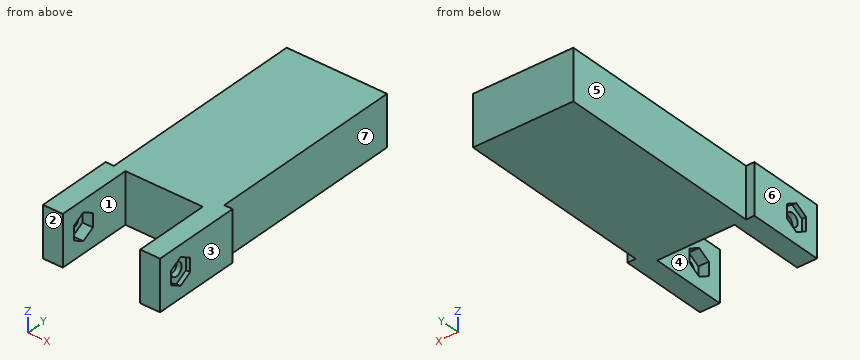
from build123d import *

# Parameters (mm, degrees)
EXTRUDE_1_DEPTH      = 12
CUT_EXTRUDE_12_DEPTH = 1
CUT_EXTRUDE_13_DEPTH = 1
CUT_EXTRUDE_14_DEPTH = 2.5
CUT_EXTRUDE_16_DEPTH = 2.5
SKETCH_26_R          = 1.55
CUT_EXTRUDE_17_DEPTH = 28


with BuildPart() as part:
    # 스케치1 → 보스-돌출1 (new body)
    with BuildSketch(Plane.XY):
        Polygon((-11.994395335, 44.774969809), (-11.994395335, -5.635030191), (-13.999795062, -5.635030191), (-13.999795062, -23.903190191), (-9.261084312, -23.903190191), (-9.261084312, -5.635030191), (9.261494188, -5.637088258), (9.261494188, -23.903190191), (14.000204938, -23.903190191), (14.000204938, -2.727088258), (12.005604665, -2.727088258), (12.005604665, 44.774969809), align=None)
    extrude(amount=EXTRUDE_1_DEPTH)

    # 스케치20 → 컷-돌출12 (cut)
    with BuildSketch(Plane(origin=(14.000204938, 0, 0), x_dir=(0, 0, -1), z_dir=(1, 0, 0))):
        Polygon((-4.384999641, -20.702278724), (-7.614999641, -20.702278724), (-9.228415158, -17.900454093), (-7.61341897, -15.106842492), (-4.380259285, -15.106842492), (-2.768420518, -17.905928971), align=None)
    extrude(amount=-CUT_EXTRUDE_12_DEPTH, mode=Mode.SUBTRACT)

    # 스케치21 → 컷-돌출13 (cut)
    with BuildSketch(Plane.ZY.offset(13.999795062)):
        Polygon((7.611047299, -20.705014823), (4.381047299, -20.705014823), (2.767631782, -17.903190191), (4.38262797, -15.109578591), (7.615787655, -15.109578591), (9.227626422, -17.90866507), align=None)
    extrude(amount=-CUT_EXTRUDE_13_DEPTH, mode=Mode.SUBTRACT)

    # 스케치22 → 컷-돌출14 (cut)
    with BuildSketch(Plane.ZY.offset(-9.261494188)):
        Polygon((7.615000359, -20.702278724), (4.385000359, -20.702278724), (2.771584842, -17.900454093), (4.38658103, -15.106842492), (7.619740715, -15.106842492), (9.231579482, -17.905928971), align=None)
    extrude(amount=-CUT_EXTRUDE_14_DEPTH, mode=Mode.SUBTRACT)

    # 스케치25 → 컷-돌출16 (cut)
    with BuildSketch(Plane(origin=(-9.261084312, 0, 0), x_dir=(0, 0, -1), z_dir=(1, 0, 0))):
        Polygon((-4.384999641, -20.702278724), (-7.614999641, -20.702278724), (-9.228415158, -17.900454093), (-7.61341897, -15.106842492), (-4.380259285, -15.106842492), (-2.768420518, -17.905928971), align=None)
    extrude(amount=-CUT_EXTRUDE_16_DEPTH, mode=Mode.SUBTRACT)

    # 스케치26 → 컷-돌출17 (cut, through all)
    with BuildSketch(Plane.ZY.offset(12.999795062)):
        with Locations((6, -17.903190191)):
            Circle(SKETCH_26_R)
    extrude(amount=-CUT_EXTRUDE_17_DEPTH, mode=Mode.SUBTRACT)


solid = part.part
The listing builds one solid part. Answer for the finished solid, in the listing's coordinates (mm). Face numbers are marked on the shaded views. A direction names the side the tool comes from. Give positions to 0.01 mm unless a question says otherwise; leave off trailing zeros. Write each loop counter-clockwise with the first axis right and the second up, starting at its lowest first coordinate (ties: lowest second). Pieces come first, ordered by that corner, then holes. Notation, with made-up numbers: (-28, 62.5) -> (10, 62.5) arc R23 ccw to (10, 80.5) -> close; hole circle Ø5 at (-18.75, -33). An arc over 180 degrees is marked (long way). Use a Markdown table: item, result.
(1) Section B-B, the plane z = 10.5 is taken. Determine the outline of the cut face in (x, y), then the cut area to 3 significant figures.
Return value:
| item | result |
|---|---|
| outline | (-14, -23.9) -> (-9.26, -23.9) -> (-9.26, -5.64) -> (9.26, -5.64) -> (9.26, -23.9) -> (14, -23.9) -> (14, -2.73) -> (12.01, -2.73) -> (12.01, 44.77) -> (-11.99, 44.77) -> (-11.99, -5.64) -> (-14, -5.64) -> close |
| area | 1,390 mm2 |
(2) For the marked faces 5, 6 and 7, determine the directions among +Z, -Z, +X, -X, +Y, -Y from which every point of the face is accessible in a straight line to the end or side of a thin tool.
Return value:
| item | result |
|---|---|
| face 5 | +Z, -Z, -X, +Y |
| face 6 | +Z, -Z, -X, +Y, -Y |
| face 7 | +Z, -Z, +X, +Y |
(3) Find the intervals of material crossed by probe 1 along Y at (x, z) = (12.4, 6); probe 2 along X at (y, z) = (-13, 1); probe 3 along Y at (x, z) = (-12.1, 6), in increasing order. Write a range as from..to.
Return value:
| item | result |
|---|---|
| probe 1 | -23.9..-19.45, -16.35..-2.73 |
| probe 2 | -14..-9.26, 9.26..14 |
| probe 3 | -23.9..-19.45, -16.35..-5.64 |
(4) Section A-A, the plane y = -12 is taken. Determine the outline of the cut face in (x, z).
Return value:
| item | result |
|---|---|
| outline | (-14, 0) -> (-9.26, 0) -> (-9.26, 12) -> (-14, 12) -> close; (9.26, 0) -> (14, 0) -> (14, 12) -> (9.26, 12) -> close |
(5) Section D-D, the plane x = -4.5 is taken. Determine the outline of the cut face in (y, z), then the cut area to 3 significant figures.
Return value:
| item | result |
|---|---|
| outline | (-5.64, 0) -> (44.77, 0) -> (44.77, 12) -> (-5.64, 12) -> close |
| area | 605 mm2 |
(6) Flat-ended cylindrical pins translate along their axes: P1, Ø0.6, axis at x = -12.5, z = 6, coming from the +Y side; P2, Ø1.5, axis at y = 35.5, z = 5.5, coming from the -X side; P3, Ø1.7, axis at y = -17.5, z = 7, coming from the +X side. Find the tip coordinate at first contact, or state that the pin passes through.
Return value:
| item | result |
|---|---|
| P1 | y = -5.64 |
| P2 | x = -11.99 |
| P3 | x = 13 |
(7) Section C-C, the plane z = 6 is taken. Give the number of separate pieces and of enclosed holes in the cut face, then the cut area to 3 significant figures.
Return value:
| item | result |
|---|---|
| separate pieces | 3 |
| enclosed holes | 0 |
| area | 1,340 mm2 |
(8) Determine the mould class of the marked faces 1, 2, 3 and 4 for opening direction X: released by +X, released by -X, zero draft, split by the parting line, or undercut.
Return value:
| item | result |
|---|---|
| face 1 | undercut |
| face 2 | zero draft |
| face 3 | released by +X |
| face 4 | undercut |
